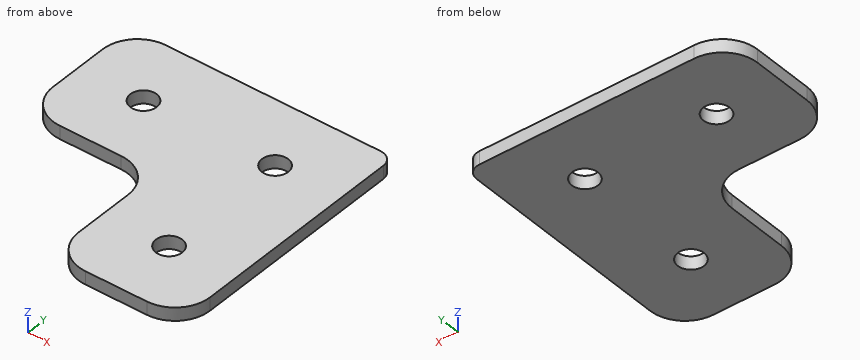
Autodesk Inventor part; units mm, degrees
ref_plane "YZ Plane" through (0, 0, 0) normal (1, 0, 0) x (0, 1, 0)
ref_plane "XZ Plane" through (0, 0, 0) normal (0, 1, 0) x (-1, 0, 0)
ref_plane "XY Plane" through (0, 0, 0) normal (0, 0, 1) x (1, 0, 0)
sketch "Szkic1" plane through (0, 0, 0) normal (0, 0, 1) x (1, 0, 0)
  line L0 (-57.3371, 37.8455) -> (-57.3371, 7.8455)
  line L1 (-57.3371, 7.8455) -> (-27.3371, 7.8455)
  line L2 (-27.3371, 7.8455) -> (-27.3371, -22.1545)
  line L3 (-27.3371, -22.1545) -> (2.6629, -22.1545)
  line L4 (2.6629, -22.1545) -> (2.6629, 37.8455)
  line L5 (2.6629, 37.8455) -> (-57.3371, 37.8455)
  point P0 (0, 0)
  point P1 (-42.3371, 22.8455)
  point P2 (-12.3371, 22.8455)
  point P3 (-12.3371, -7.1545)
  dimension "d0" = 30
  dimension "d1" = 30
  dimension "d2" = 30
  dimension "d3" = 30
  dimension "d4" = 15
  dimension "d5" = 15
  dimension "d6" = 15
  dimension "d7" = 15
  dimension "d8" = 15
  dimension "d9" = 15
extrude "Wyciągnięcie proste1" add sketch "Szkic1" along normal blind 3
hole "Otwór1" at (-42.3371, 22.8455, 0) at (-12.3371, 22.8455, 0) at (-12.3371, -7.1545, 0) direction (0, 0, 1) diameter 6 end through all
fillet "Zaokrąglenie2" radius 3 1 edges at (2.6629, 37.8455, 1.5)
fillet "Zaokrąglenie3" radius 8 5 edges at (2.6629, -22.1545, 1.5) (-27.3371, -22.1545, 1.5) (-27.3371, 7.8455, 1.5) (-57.3371, 7.8455, 1.5) (-57.3371, 37.8455, 1.5)
equation "\"d1\" = d0"
equation "\"d3\" = d2"
properties part number "LC_ALU_3mm_30x30_Corner_Bracket"
The listing builds one solid part. Answer for the finished solid, in the listing's coordinates (mm). Coordinates: 2 decimals unless noted, no trailing zeros. Write each loop counter-clockwise with the first axis right and the second up, starting at its lowest first coordinate (ties: lowest second). Pieces come first, ordered by that corner, then holes. Notation, with made-up numbers: M 40.5,27 L 65.5,27 A9 ccw 65.5,33 Z; hole C 8.5,86 d3. An arc over 180 degrees is marked long. Use one line per item in the form item = value.
Item 1: Find the intervals of material crossed by probe 1 along Y at (x, z) = (-10.5, 0.4); probe 2 along Y at (x, z) = (-42.5, 0.5); probe 3 along X at (y, z) = (15.5, 2.1), in increasing order.
Model answer:
probe_1 = -22.15 to -9.53, -4.78 to 20.47, 25.22 to 37.85
probe_2 = 7.85 to 19.85, 25.84 to 37.85
probe_3 = -57.33 to 2.66
Item 2: Find section A-A, the plane y = 24. Give the vertices of the cut face in (x, z), plus the area to 3 significant figures.
Model answer:
outline = M -57.34,0 L -45.11,0 L -45.11,3 L -57.34,3 Z; M -39.57,0 L -15.11,0 L -15.11,3 L -39.57,3 Z; M -9.57,0 L 2.66,0 L 2.66,3 L -9.57,3 Z
area = 147 mm2
Item 3: Given P1, Ø5, axis at x = -42.34, y = 22.85, coming from the -Z side, flat-ended and moving along its own axis, determine where the tip first touches the part or whether it passes through.
Model answer:
P1 = through
Item 4: Find section D-D, the plane x = -47.5. Give the vertices of the cut face in (y, z), plus the area to 3 significant figures.
Model answer:
outline = M 7.85,0 L 37.85,0 L 37.85,3 L 7.85,3 Z
area = 90.0 mm2
Item 5: Find section B-B, the plane z = 2.45. Give the vertices of the cut face in (x, y).
Model answer:
outline = M -57.34,15.85 A8 ccw -49.34,7.85 L -35.34,7.85 A8 cw -27.34,-0.15 L -27.34,-14.15 A8 ccw -19.34,-22.15 L -5.34,-22.15 A8 ccw 2.66,-14.15 L 2.66,34.85 A3 ccw -0.34,37.85 L -49.34,37.85 A8 ccw -57.34,29.85 Z; hole C -42.34,22.85 d6; hole C -12.34,-7.15 d6; hole C -12.34,22.85 d6
Item 6: Find section C-C, the plane y = -6.5. Give the vertices of the cut face in (x, z).
Model answer:
outline = M -27.34,0 L -15.26,0 L -15.26,3 L -27.34,3 Z; M -9.41,0 L 2.66,0 L 2.66,3 L -9.41,3 Z
